```python
from build123d import *

# Parameters (mm, degrees)
SKETCH2_R              = 1.4
SKETCH2_R_2            = 30
BOSS_EXTRUDE1_DEPTH    = 5
SKETCH3_R              = 3.2
BOSS_EXTRUDE2_DEPTH    = 5
SKETCH5_W              = 15.2
SKETCH5_H              = 25
CUT_EXTRUDE2_DEPTH     = 152.952036544
SKETCH7_R              = 1.4
SKETCH7_R_2            = 1.5
SKETCH7_W              = 25
SKETCH7_H              = 8
CUT_EXTRUDE3_DEPTH     = 152.952036544
BOSS_EXTRUDE3_DEPTH    = 5
CUT_EXTRUDE4_OUTLINE_R = 1.4
CUT_EXTRUDE4_DEPTH     = 5
CUT_EXTRUDE5_DEPTH     = 181.884990958
FILLET1_R              = 5
FILLET2_R              = 20
FILLET3_R              = 2


# Read off the part's stored shape, not the designer's step: Cut-Extrude4
with BuildPart() as part:
    # Sketch2 → Boss-Extrude1 (new body)
    with BuildSketch(Plane(origin=(0, 0, 0), x_dir=(1, 0, 0), z_dir=(0, 1, 0))):
        Polygon((46.354723211, 80.288735773), (-46.354723211, 80.288735773), (-92.709446423, 0), (-46.354723211, -80.288735773), (46.354723211, -80.288735773), (92.709446423, 0), align=None)
        with Locations(Location((26, 69.288735773, 0), (0, 0, 270))):
            Circle(SKETCH2_R, mode=Mode.SUBTRACT)
        with Locations(Location((26, 49.288735773, 0), (0, 0, 270))):
            Circle(SKETCH2_R, mode=Mode.SUBTRACT)
        with Locations(Location((-26, 49.288735773, 0), (0, 0, 270))):
            Circle(SKETCH2_R, mode=Mode.SUBTRACT)
        with Locations(Location((-26, 69.288735773, 0), (0, 0, 270))):
            Circle(SKETCH2_R, mode=Mode.SUBTRACT)
        with Locations(Location((0, 0, 0), (0, 0, 270))):
            Circle(SKETCH2_R_2, mode=Mode.SUBTRACT)
        with Locations(Location((55.6852973, -2.127707388, 0), (0, 0, 270))):
            Circle(SKETCH2_R, mode=Mode.SUBTRACT)
        with Locations(Location((73.005805376, -12.127707388, 0), (0, 0, 270))):
            Circle(SKETCH2_R, mode=Mode.SUBTRACT)
        with Locations(Location((47.005805376, -57.161028385, 0), (0, 0, 270))):
            Circle(SKETCH2_R, mode=Mode.SUBTRACT)
        with Locations(Location((29.6852973, -47.161028385, 0), (0, 0, 270))):
            Circle(SKETCH2_R, mode=Mode.SUBTRACT)
        with Locations(Location((-29.6852973, -47.161028385, 0), (0, 0, 270))):
            Circle(SKETCH2_R, mode=Mode.SUBTRACT)
        with Locations(Location((-47.005805376, -57.161028385, 0), (0, 0, 270))):
            Circle(SKETCH2_R, mode=Mode.SUBTRACT)
        with Locations(Location((-73.005805376, -12.127707388, 0), (0, 0, 270))):
            Circle(SKETCH2_R, mode=Mode.SUBTRACT)
        with Locations(Location((-55.6852973, -2.127707388, 0), (0, 0, 270))):
            Circle(SKETCH2_R, mode=Mode.SUBTRACT)
    extrude(amount=BOSS_EXTRUDE1_DEPTH)

    # Sketch3 → Boss-Extrude2 (add)
    with BuildSketch(Plane(origin=(0, 0, 0), x_dir=(1, 0, 0), z_dir=(0, 1, 0))):
        Polygon((46.354723211, 120.288735773), (92.709446423, 120.288735773), (92.709446423, 0), (46.354723211, 80.288735773), (-46.354723211, 80.288735773), align=None)
        with Locations(Location((71.203193978, 100.288735773, 0), (0, 0, 270))):
            Circle(SKETCH3_R, mode=Mode.SUBTRACT)
    extrude(amount=BOSS_EXTRUDE2_DEPTH)

    # Sketch5 → Cut-Extrude2 (cut, through all)
    with BuildSketch(Plane(origin=(0, 5, 0), x_dir=(1, 0, 0), z_dir=(0, 1, 0))):
        with Locations((0, -41.521371436)):
            Rectangle(SKETCH5_W, SKETCH5_H)
    extrude(amount=-CUT_EXTRUDE2_DEPTH, mode=Mode.SUBTRACT)

    # Sketch7 → Cut-Extrude3 (cut, through all)
    with BuildSketch(Plane.XZ):
        with Locations(Location((-12.5, 39.021371436, 0), (0, 0, 270))):
            Circle(SKETCH7_R)
        with Locations(Location((12.5, 39.021371436, 0), (0, 0, 270))):
            Circle(SKETCH7_R)
        with Locations((-6.539339828, 52.960711264)):
            Circle(SKETCH7_R_2)
        with Locations((6.539339828, 52.960711264)):
            Circle(SKETCH7_R_2)
        with Locations((0, 31.271780287)):
            Rectangle(SKETCH7_W, SKETCH7_H)
    extrude(amount=-CUT_EXTRUDE3_DEPTH, mode=Mode.SUBTRACT)

    # Sketch8 → Boss-Extrude3 (add)
    with BuildSketch(Plane(origin=(0, 0, 0), x_dir=(1, 0, 0), z_dir=(0, 1, 0))):
        Polygon((-92.709446423, 0), (-135, 0), (-135, 80.288735773), (-46.354723211, 80.288735773), align=None)
        Polygon((92.709446423, 0), (135, 0), (135, 80.288735773), (92.709446423, 120.288735773), align=None)
    extrude(amount=BOSS_EXTRUDE3_DEPTH)

    # Cut-Extrude4 outline → Cut-Extrude4 (cut)
    with BuildSketch(Plane(origin=(0, 0, 0), x_dir=(1, 0, 0), z_dir=(0, 1, 0))):
        with Locations((-37.601356721, 60.891621456)):
            Circle(CUT_EXTRUDE4_OUTLINE_R)
        with Locations((-127.5, 66.288735773)):
            Circle(CUT_EXTRUDE4_OUTLINE_R)
        with Locations((-127.5, 15.498735773)):
            Circle(CUT_EXTRUDE4_OUTLINE_R)
        with Locations((127.5, 15.5)):
            Circle(CUT_EXTRUDE4_OUTLINE_R)
        with Locations((-59.251991815, 73.391621456)):
            Circle(CUT_EXTRUDE4_OUTLINE_R)
        with Locations((-84.251991815, 30.090351267)):
            Circle(CUT_EXTRUDE4_OUTLINE_R)
        with Locations((-62.601356721, 17.590351267)):
            Circle(CUT_EXTRUDE4_OUTLINE_R)
        with Locations((127.5, 66.29)):
            Circle(CUT_EXTRUDE4_OUTLINE_R)
    extrude(amount=CUT_EXTRUDE4_DEPTH, mode=Mode.SUBTRACT)

    # Sketch10 → Cut-Extrude5 (cut, through all)
    with BuildSketch(Plane(origin=(0, 5, 0), x_dir=(1, 0, 0), z_dir=(0, 1, 0))):
        Polygon((-46.354723211, 80.288735773), (135, 80.288735773), (92.709446423, 120.288735773), (46.354723211, 120.288735773), align=None)
    extrude(amount=-CUT_EXTRUDE5_DEPTH, mode=Mode.SUBTRACT)

    # Fillet1
    fillet1_edges = [part.edges().sort_by_distance(p)[0] for p in [
        (46.354723211, 2.5, 80.288735773),
        (-46.354723211, 2.5, 80.288735773),
        (-135, 2.5, -80.288735773),
        (-135, 2.5, 0),
        (135, 2.5, 0),
        (135, 2.5, -80.288735773),
    ]]
    fillet(fillet1_edges, radius=FILLET1_R)

    # Fillet2
    fillet2_edges = [part.edges().sort_by_distance(p)[0] for p in [
        (92.709446423, 2.5, 0),
        (-92.709446423, 2.5, 0),
    ]]
    fillet(fillet2_edges, radius=FILLET2_R)

    # Fillet3
    fillet3_edges = [part.edges().sort_by_distance(p)[0] for p in [
        (7.6, 2.5, 35.271780287),
        (-7.6, 2.5, 35.271780287),
        (-12.5, 2.5, 35.271780287),
        (12.5, 2.5, 35.271780287),
        (12.5, 2.5, 27.271780287),
        (-12.5, 2.5, 27.271780287),
    ]]
    fillet(fillet3_edges, radius=FILLET3_R)


solid = part.part
```
Here's how the part is built. I have some questions about the finished solid (model axes, mm). A direction names the side the tool comes from. Coordinates: 2 decimals unless noted, no trailing zeros. Write each loop counter-clockwise with the first axis right and the second up, starting at its lowest first coordinate (ties: lowest second). Pieces come first, ordered by that corner, then holes. Notation, with made-up numbers: (88.5, 63) -> (121.5, 63) arc R15 cw to (121.5, 68) -> close; hole circle Ø7 at (10.5, -30.5). An arc over 180 degrees is marked (long way). Use a Markdown table: item, result. Add a question column.
(1) Please list where these lines run through material, in increasing order: line 1 (X direction, y = 2.55, z = -67.5); line 2 (Z direction, x = 0, y = 2.2); line 3 (X direction, y = 4.5, z = 12.5).
(2) For faces 4 (the flat face through (-7.6, 3, 45)), 5 (the flat face through (2, 0, -37)), 6 (the flat face through (-117, 2, 0)), which set-ups out of +Z, -Z, +X, -X, +Y, -Y let a thin tool reach every point of the face, with its end or its side?
(3) If we section it at B-B, the plane z = 21.5: Write out the boundary of the cut face in (x, y).
(4) We'd pull the mould along Z, two halves only. Please class faces 1 (the cylindrical face through (94.13, 2.535, 2.753)), 2 (the cylindrical face through (133.57, 2.54, -78.79)), 3 (the flat face through (0, 3, 54.021)): +Z half, -Z half, draft (parallel to the pull), parting line (faces both ways), or undercut.
(5) If we section it at A-A, the plane x = 0: Write out the boundary of the cut face in (y, z).
(6) If we section it at D-D, the plane y = 1.8: State how many separate pieces and enclosed holes the cut face has, and give its area (3 significant figures).
(7) I'm going to push flat-ended pins straight in: P1, Ø1.5, axis at x = -48.5, y = 1.5, coming from the +Z side; P2, Ø1, axis at y = 1, z = 25.5, coming from the -X side. Where does each tip first touch, or does it pass through?
(8) If we section it at C-C, the plane x = 115: Write out the boundary of the cut face in (y, z), and give its area (3 significant figures).
Outcome:
| question | item | result |
|---|---|---|
| 1 | line 1 | x = -135 to -128.2, -126.8 to 126.8, 128.2 to 135 |
| 1 | line 2 | z = -80.29 to -30, 54.02 to 80.29 |
| 1 | line 3 | x = -85.49 to -74.36, -71.66 to -27.27, 27.27 to 71.66, 74.36 to 85.49 |
| 2 | face 4 | +Y, -Y |
| 2 | face 5 | +Z, -Z, +X, -X, -Y |
| 2 | face 6 | +Z, -X, +Y, -Y |
| 3 | outline | (-80.3, 0) -> (-20.92, 0) -> (-20.92, 5) -> (-80.3, 5) -> close; (20.92, 0) -> (80.3, 0) -> (80.3, 5) -> (20.92, 5) -> close |
| 4 | face 1 | +Z half |
| 4 | face 2 | -Z half |
| 4 | face 3 | undercut |
| 5 | outline | (0, -80.29) -> (5, -80.29) -> (5, -30) -> (0, -30) -> close; (0, 54.02) -> (5, 54.02) -> (5, 80.29) -> (0, 80.29) -> close |
| 6 | separate pieces | 1 |
| 6 | enclosed holes | 23 |
| 6 | area | 29,500 mm^2 |
| 7 | P1 | stops at z = 77.87 |
| 7 | P2 | stops at x = -78.28 |
| 8 | outline | (0, -80.29) -> (5, -80.29) -> (5, 0) -> (0, 0) -> close |
| 8 | area | 401 mm^2 |
